Geometry: final body of the model. Coordinates: model frame, mm. Face numbers are marked on the shaded views. A direction names the side the tool comes from. Round coordinates to 2 decimals unless told otherwise and drop trailing zeros. Loops run counter-clockwise (first coordinate to the right, second up) from the corner with the lowest first, then second, coordinate; pieces in that order, holes last. Notation, with made-up numbers: (57, 76) -> (91, 76) arc R13 cw to (91, 86) -> close; hole circle Ø7 at (19.25, -2). An arc over 180 degrees is marked (long way). Answer in a Markdown table with one row per item.
```python
from build123d import *

# Parameters (mm, degrees)
SKETCH1_R           = 10
SKETCH1_R_2         = 1.6
BOSS_EXTRUDE1_DEPTH = 2
SKETCH1_3_R         = 1.3
BOSS_EXTRUDE2_DEPTH = 4
CHAMFER1_SIZE       = 1
SKETCH1_5_R         = 2.3
SKETCH1_5_R_2       = 1.6
BOSS_EXTRUDE4_DEPTH = 7.5


with BuildPart() as part:
    # Sketch1 → Boss-Extrude1 (new body)
    with BuildSketch(Plane.XY):
        Circle(SKETCH1_R)
        Circle(SKETCH1_R_2, mode=Mode.SUBTRACT)
    extrude(amount=BOSS_EXTRUDE1_DEPTH)

    # Sketch1_3 → Boss-Extrude2 (add)
    with BuildSketch(Plane.XY):
        with Locations((-5.5, 5.5)):
            Circle(SKETCH1_3_R)
        with Locations((5.5, 5.5)):
            Circle(SKETCH1_3_R)
        with Locations((5.5, -5.5)):
            Circle(SKETCH1_3_R)
        with Locations((-5.5, -5.5)):
            Circle(SKETCH1_3_R)
    extrude(amount=-BOSS_EXTRUDE2_DEPTH)

    # Chamfer1
    chamfer1_edges = [part.edges().sort_by_distance(p)[0] for p in [
        (-10, 0, 2),
    ]]
    chamfer(chamfer1_edges, length=CHAMFER1_SIZE)

    # Sketch1_5 → Boss-Extrude4 (add)
    with BuildSketch(Plane.XY):
        Circle(SKETCH1_5_R)
        Circle(SKETCH1_5_R_2, mode=Mode.SUBTRACT)
    extrude(amount=-BOSS_EXTRUDE4_DEPTH)


solid = part.part
```
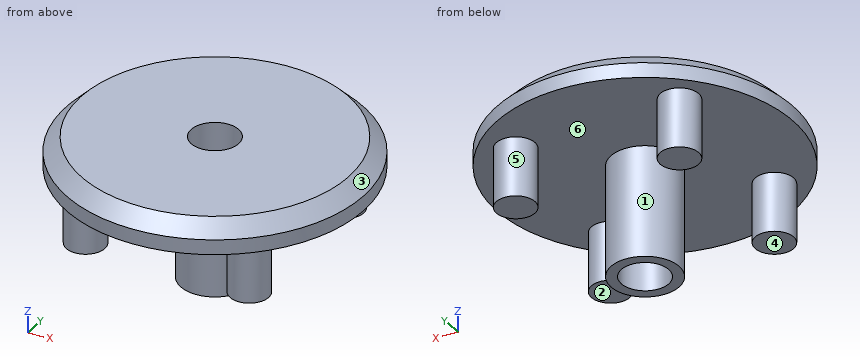
Item 1: First-contact query: P1, Ø1.3, axis at x = 5.5, y = -5.5, coming from the -Z side; P2, Ø4, axis at x = 6, z = -3.5, coming from the +Y side; P3, Ø3, axis at x = 0, z = -5, coming from the -Y side; P4, Ø1.9, axis at x = 0, y = 0, coming from the +Z side (3 decimals). Flat tips, straight axial feed; report the tip coordinate or a pass-through.
Ans:
| item | result |
|---|---|
| P1 | z = -4 |
| P2 | y = 6.8 |
| P3 | y = -2.3 |
| P4 | through |
Item 2: Section query B-B, the plane x = 0. Output: boundary loops of the cut face in (y, z), and give its area (3 significant figures).
Ans:
| item | result |
|---|---|
| outline | (-10, 0) -> (-2.3, 0) -> (-2.3, -7.5) -> (-1.6, -7.5) -> (-1.6, 2) -> (-9, 2) -> (-10, 1) -> close; (1.6, -7.5) -> (2.3, -7.5) -> (2.3, 0) -> (10, 0) -> (10, 1) -> (9, 2) -> (1.6, 2) -> close |
| area | 43.1 mm2 |
Item 3: Set-up query: the marked faces 1 and 2. Return all of +Z, -Z, +X, -X, +Y, -Y with unobstructed straight access to the full face (end or side cutting, diameter ignored); none if empty.
Ans:
| item | result |
|---|---|
| face 1 | -Z |
| face 2 | -Z, +X, -X, +Y, -Y |
Item 4: Section query C-C, the plane z = 1.75. Output: boundary loops of the cut face in (x, y).
Ans:
| item | result |
|---|---|
| outline | circle Ø18.5 at (0, 0); hole circle Ø3.2 at (0, 0) |
Item 5: Ray query, L1, parallel to Y at x = 0, z = -5.25; L2, parallel to Y at x = 0, z = 0.7; L3, parallel to Z at x = 8, y = -1.75. Return the intervals inside material, ascending.
Ans:
| item | result |
|---|---|
| L1 | -2.3 to -1.6, 1.6 to 2.3 |
| L2 | -10 to -1.6, 1.6 to 10 |
| L3 | 0 to 2 |
Item 6: Section query A-A, the plane z = -1.25. Output: boundary loops of the cut face in (x, y), and give its area (3 significant figures).
Ans:
| item | result |
|---|---|
| outline | circle Ø2.6 at (-5.5, -5.5); circle Ø2.6 at (-5.5, 5.5); circle Ø4.6 at (0, 0); circle Ø2.6 at (5.5, -5.5); circle Ø2.6 at (5.5, 5.5); hole circle Ø3.2 at (0, 0) |
| area | 29.8 mm2 |
Item 7: Mould query, pull axis Y, two halves, no side actions, for the marked faces 3, 4, 5 and 6. Classes: released by +Y, released by -Y, zero draft, split by the parting line, or undercut.
Ans:
| item | result |
|---|---|
| face 3 | split by the parting line |
| face 4 | zero draft |
| face 5 | undercut |
| face 6 | undercut |
